For this review, take the finished solid that the model builds, in its own axes (mm). A direction names the side the tool comes from. Give positions to 0.01 mm unless a question says otherwise; leave off trailing zeros. Write each loop counter-clockwise with the first axis right and the second up, starting at its lowest first coordinate (ties: lowest second). Pieces come first, ordered by that corner, then holes. Notation, with made-up numbers: (84, 54.25) -> (119, 54.25) arc R14 ccw to (119, 60.25) -> close; hole circle Ø10 at (-31.5, 58). An arc over 180 degrees is marked (long way). Return JSON: item names as keys, results as strings.
from build123d import *

# Parameters (mm, degrees)
BOSS_EXTRUDE1_DEPTH      = 2
SKETCH2_W                = 2
SKETCH2_H                = 60
BOSS_EXTRUDE2_DEPTH      = 55
SKETCH3_R                = 5
CUT_EXTRUDE1_DEPTH       = 283
SKETCH4_R                = 2.5
CUT_EXTRUDE2_DEPTH       = 283
SKETCH9_W                = 230
SKETCH9_H                = 50
BOSS_EXTRUDE3_DEPTH      = 2
SKETCH13_W               = 230
SKETCH13_H               = 10
BOSS_EXTRUDE6_DEPTH      = 20
CUT_EXTRUDE9_START       = -230
CUT_EXTRUDE9_DEPTH       = 230
SKETCH31_R               = 2.5
CUT_EXTRUDE11_DEPTH      = 10
SKETCH32_R               = 2.5
CUT_EXTRUDE12_DEPTH      = 10
SKETCH33_R               = 2.5
CUT_EXTRUDE13_DEPTH      = 10
CUT_EXTRUDE14_DEPTH      = 180.947909129
CUT_EXTRUDE14_DEPTH_BACK = 180.947909129
CUT_EXTRUDE16_DEPTH      = 151.685931659
CUT_EXTRUDE16_DEPTH_BACK = 151.685931659
BOSS_EXTRUDE8_DEPTH      = 60


# Read off the part's stored shape, not the designer's step: Cut-Extrude9
with BuildPart() as part:
    # Sketch1 → Boss-Extrude1 (new body)
    with BuildSketch(Plane(origin=(0, 0, 0), x_dir=(1, 0, 0), z_dir=(0, 1, 0))):
        Polygon((115, 50), (115, 80), (-115, 80), (-115, 50), (-115, -50), (-115, -75), (115, -75), (115, -50), align=None)
    extrude(amount=BOSS_EXTRUDE1_DEPTH)

    # Sketch2 → Boss-Extrude2 (add)
    with BuildSketch(Plane(origin=(0, 2, 0), x_dir=(1, 0, 0), z_dir=(0, 1, 0))):
        with Locations((-114, 0)):
            Rectangle(SKETCH2_W, SKETCH2_H)
        with Locations((114, 0)):
            Rectangle(SKETCH2_W, SKETCH2_H)
    extrude(amount=BOSS_EXTRUDE2_DEPTH)

    # Sketch3 → Cut-Extrude1 (cut)
    with BuildSketch(Plane.ZY.offset(115)):
        with Locations((0, 29.5)):
            Circle(SKETCH3_R)
    extrude(amount=-CUT_EXTRUDE1_DEPTH, mode=Mode.SUBTRACT)

    # Sketch4 → Cut-Extrude2 (cut)
    with BuildSketch(Plane.ZY.offset(115)):
        with Locations((-22.5, 29.5)):
            Circle(SKETCH4_R)
        with Locations((22.5, 29.5)):
            Circle(SKETCH4_R)
    extrude(amount=-CUT_EXTRUDE2_DEPTH, mode=Mode.SUBTRACT)

    # Sketch9 → Boss-Extrude3 (add)
    with BuildSketch(Plane(origin=(0, 2, 0), x_dir=(1, 0, 0), z_dir=(0, 1, 0))):
        with Locations((0, 105)):
            Rectangle(SKETCH9_W, SKETCH9_H)
    extrude(amount=-BOSS_EXTRUDE3_DEPTH)

    # Sketch13 → Boss-Extrude6 (add)
    with BuildSketch(Plane.XZ):
        with Locations((0, -125)):
            Rectangle(SKETCH13_W, SKETCH13_H)
    extrude(amount=BOSS_EXTRUDE6_DEPTH)

    # Cut-Extrude9 outline → Cut-Extrude9 (cut)
    with BuildSketch(Plane(origin=(115, 0, 0), x_dir=(0, 0, -1), z_dir=(1, 0, 0)).offset(CUT_EXTRUDE9_START)):
        with BuildLine():
            Line((-30, 57), (-30, 29.5))
            ThreePointArc((-30, 29.5), (0, 49.5), (30, 29.5))
            Line((30, 29.5), (30, 57))
            Line((30, 57), (-30, 57))
        make_face()
    extrude(amount=CUT_EXTRUDE9_DEPTH, mode=Mode.SUBTRACT)

    # Sketch31 → Cut-Extrude11 (cut)
    with BuildSketch(Plane(origin=(0, 2, 0), x_dir=(1, 0, 0), z_dir=(0, 1, 0))):
        with Locations(Location((-27.5, 65, 0), (0, 0, 270))):
            Circle(SKETCH31_R)
        with Locations(Location((27.5, 65, 0), (0, 0, 270))):
            Circle(SKETCH31_R)
        with Locations(Location((-27.5, 25, 0), (0, 0, 270))):
            Circle(SKETCH31_R)
        with Locations(Location((27.5, 25, 0), (0, 0, 270))):
            Circle(SKETCH31_R)
    extrude(amount=-CUT_EXTRUDE11_DEPTH, mode=Mode.SUBTRACT)

    # Sketch32 → Cut-Extrude12 (cut)
    with BuildSketch(Plane(origin=(0, 2, 0), x_dir=(1, 0, 0), z_dir=(0, 1, 0))):
        with Locations(Location((85, 70, 0), (0, 0, 270))):
            Circle(SKETCH32_R)
        with Locations(Location((65, 70, 0), (0, 0, 270))):
            Circle(SKETCH32_R)
        with Locations(Location((65, 20, 0), (0, 0, 90))):
            Circle(SKETCH32_R)
        with Locations(Location((85, 20, 0), (0, 0, 90))):
            Circle(SKETCH32_R)
    extrude(amount=-CUT_EXTRUDE12_DEPTH, mode=Mode.SUBTRACT)

    # Sketch33 → Cut-Extrude13 (cut)
    with BuildSketch(Plane(origin=(0, 2, 0), x_dir=(1, 0, 0), z_dir=(0, 1, 0))):
        with Locations(Location((-20, 10.45, 0), (0, 0, 270))):
            Circle(SKETCH33_R)
        with Locations(Location((20, 10.45, 0), (0, 0, 270))):
            Circle(SKETCH33_R)
        with Locations(Location((-20, -29.55, 0), (0, 0, 270))):
            Circle(SKETCH33_R)
        with Locations(Location((20, -29.55, 0), (0, 0, 90))):
            Circle(SKETCH33_R)
    extrude(amount=-CUT_EXTRUDE13_DEPTH, mode=Mode.SUBTRACT)

    # Sketch34 → Cut-Extrude14 (cut, two sides: drawn at the far end of the back side and taken through both)
    with BuildSketch(Plane(origin=(0, 2, 0), x_dir=(1, 0, 0), z_dir=(0, 1, 0)).offset(-CUT_EXTRUDE14_DEPTH_BACK)):
        Polygon((685.357029045, 85), (115, 85), (-115, 85), (-685.357029045, 85), (-685.357029045, 1225.71405809), (685.357029045, 1225.71405809), align=None)
    extrude(amount=CUT_EXTRUDE14_DEPTH + CUT_EXTRUDE14_DEPTH_BACK, mode=Mode.SUBTRACT)

    # Sketch36 → Cut-Extrude16 (cut, two sides: drawn at the far end of the back side and taken through both)
    with BuildSketch(Plane(origin=(0, 2, 0), x_dir=(1, 0, 0), z_dir=(0, 1, 0)).offset(-CUT_EXTRUDE16_DEPTH_BACK)):
        with BuildLine():
            Line((-603.246524362, 161.052987794), (-115, -30))
            Line((-115, -30), (-7.287986972, -72.148179011))
            ThreePointArc((-7.287986972, -72.148179011), (0, -73.523323417), (7.287986972, -72.148179011))
            Line((7.287986972, -72.148179011), (115, -30))
            Line((115, -30), (603.246524362, 161.052987794))
            Line((603.246524362, 161.052987794), (603.246524362, -887.538281856))
            Line((603.246524362, -887.538281856), (-603.246524362, -887.538281856))
            Line((-603.246524362, -887.538281856), (-603.246524362, 161.052987794))
        make_face()
    extrude(amount=CUT_EXTRUDE16_DEPTH + CUT_EXTRUDE16_DEPTH_BACK, mode=Mode.SUBTRACT)

    # Sketch37 → Boss-Extrude8 (add)
    with BuildSketch(Plane(origin=(0, 0, -30), x_dir=(-1, 0, 0), z_dir=(0, 0, -1))):
        with BuildLine():
            Line((-103, 2), (-113, 2))
            Line((-113, 2), (-113, 12))
            ThreePointArc((-113, 12), (-110.071067812, 4.928932188), (-103, 2))
        make_face()
        with BuildLine():
            Line((103, 2), (113, 2))
            Line((113, 2), (113, 12))
            ThreePointArc((113, 12), (110.071067812, 4.928932188), (103, 2))
        make_face()
    extrude(amount=-BOSS_EXTRUDE8_DEPTH)


solid = part.part
1. Add section D-D, the plane z = -65. State the section outline as (x, y) points, plus the area to 3 significant figures.
Results found:
{"outline": "(-115, 0) -> (-30, 0) -> (-30, 2) -> (-115, 2) -> close; (-25, 0) -> (25, 0) -> (25, 2) -> (-25, 2) -> close; (30, 0) -> (115, 0) -> (115, 2) -> (30, 2) -> close", "area": "440 mm²"}
2. Add section A-A, the plane z = 0. State the section outline as (x, y) points.
Results found:
{"outline": "(-115, 0) -> (115, 0) -> (115, 24.5) -> (113, 24.5) -> (113, 12) arc R10 cw to (103, 2) -> (-103, 2) arc R10 cw to (-113, 12) -> (-113, 24.5) -> (-115, 24.5) -> close; (-115, 34.5) -> (-113, 34.5) -> (-113, 49.5) -> (-115, 49.5) -> close; (113, 34.5) -> (115, 34.5) -> (115, 49.5) -> (113, 49.5) -> close"}
3. To check wall thickness, follow probe 1 along X at (y, z) = (1.2, -10.45); probe 2 along X at (y, z) = (0.7, -20); probe 3 along X at (y, z) = (21, 3.5). State the ranges of each line that lie inside material, in increasing order.
Results found:
{"probe 1": "x = -115 to -22.5, -17.5 to 17.5, 22.5 to 115", "probe 2": "x = -115 to 62.5, 67.5 to 82.5, 87.5 to 115", "probe 3": "x = -115 to -113, 113 to 115"}
4. The part is to be moulded in two halves that separate along Y. For faces 4 (the cylindrical face through (113.99, 31.19, 20.66)), 5 (the cylindrical face through (-110.15, 5.01, -0.42)), 6 (the cylindrical face through (29.61, 1.01, -63.66)), 7 (the cylindrical face through (-114.01, 31.19, -24.34)), say which applies: +Y half, -Y half, draft (parallel to the pull), parting line (faces both ways), or undercut.
Results found:
{"face 4": "undercut", "face 5": "+Y half", "face 6": "draft", "face 7": "undercut"}
5. For pin 1 (8 mm diameter, centred on x = 16.5, z = 8.5, fed in from +Y), flat-tipped, find the tip position at first contact; note if it passes through.
Results found:
{"pin 1": "stops at y = 2"}
6. Add section C-C, the plane y = 38. State the section outline as (x, z) points, plus the area to 3 significant figures.
Results found:
{"outline": "(-115, -24.8) -> (-113, -24.8) -> (-113, 24.8) -> (-115, 24.8) -> close; (113, -24.8) -> (115, -24.8) -> (115, 24.8) -> (113, 24.8) -> close", "area": "198 mm²"}
7. For faces 1 (the flat face through (-113, 22, 0)), 2 (the flat face through (-113.5, 12.6, 30)), 3 (the flat face through (60.39, 0.99, 51.37)), list the 3-axis set-ups (+Z, -Z, +X, -X, +Y, -Y) from which the entire face can be reached by the end or side of a thin tool; tool diameter is ignored.
Results found:
{"face 1": "+Z, -Z, +Y", "face 2": "+Z, +X, -X, +Y", "face 3": "+Z, +X, +Y, -Y"}
8. Add section B-B, the plane x = 65. State the section outline as (y, z) points, plus the area to 3 significant figures.
Results found:
{"outline": "(0, -85) -> (2, -85) -> (2, -72.5) -> (0, -72.5) -> close; (0, -67.5) -> (2, -67.5) -> (2, -22.5) -> (0, -22.5) -> close; (0, -17.5) -> (2, -17.5) -> (2, 49.57) -> (0, 49.57) -> close", "area": "249 mm²"}
